Drawing for the job (mm, zero at the part's lowest x, y, z). A direction names the side the tool comes from. Coordinates: 2 decimals unless noted, no trailing zeros. Loops run counter-clockwise (first coordinate to the right, second up) from the corner with the lowest first, then second, coordinate; pieces in that order, holes last. Notation, with made-up numbers: (65, -16.5) -> (76, -16.5) arc R14 cw to (76, -11.5) -> close; hole circle Ø11 at (70.5, 57.5). An arc over 180 degrees is marked (long way). Write each question's results on one line, items separated by ' | '.
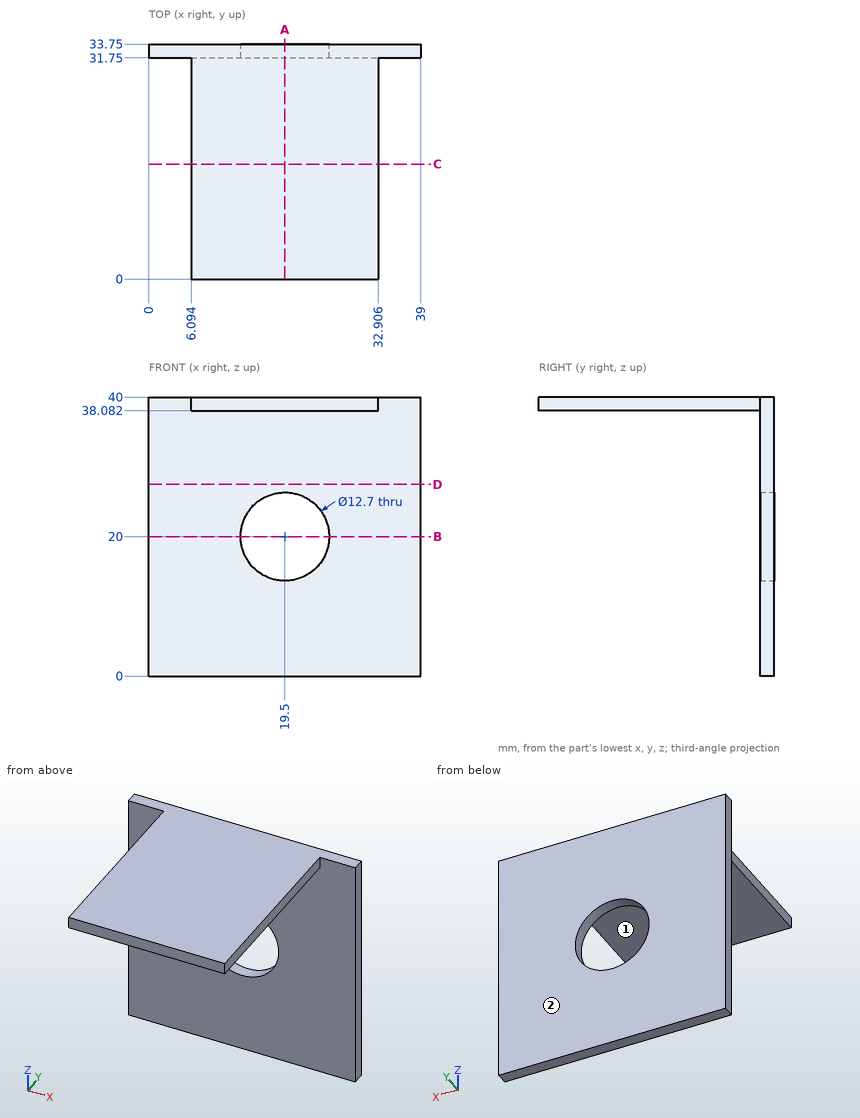
1) Slice it at A-A (x = 19.5). Write the cut outline in (y, z).
Outcome:
outline: (0, 38.08) -> (31.75, 38.08) -> (31.75, 26.35) -> (33.75, 26.35) -> (33.75, 40) -> (0, 40) -> close; (31.75, 0) -> (33.75, 0) -> (33.75, 13.65) -> (31.75, 13.65) -> close
2) Slice it at D-D (z = 27.5). Write the cut outline in (x, y), then the cut area to 3 significant figures.
Outcome:
outline: (0, 31.75) -> (39, 31.75) -> (39, 33.75) -> (0, 33.75) -> close | area: 78.0 mm^2
3) Slice it at C-C (y = 16.5). Write the cut outline in (x, z).
Outcome:
outline: (6.09, 38.08) -> (32.91, 38.08) -> (32.91, 40) -> (6.09, 40) -> close
4) Pin check, flat tips, straight feed: pin 1 (10 mm diameter, centred on y = 28, z = 14, fed in from -X); pin 2 (2 mm diameter, centred on y = 29.5, z = 32, fed in from -X); pin 3 (16.5 mm diameter, centred on x = 19.5, z = 20, fed in from -Y); pin 4 (8 mm diameter, centred on x = 26, y = 15.5, fed in from -Z). Stop position of each tip, or through.
Outcome:
pin 1: stops at x = 0 | pin 2: passes through | pin 3: stops at y = 31.75 | pin 4: stops at z = 38.08
5) Which spindle directions (+Z, -Z, +X, -X, +Y, -Y) get a long thin tool onto all of the face, cutting with end or side? Do the marked faces 1 and 2. Say none if no direction does.
Outcome:
face 1: -Z, +X, -X, -Y | face 2: +Z, -Z, +X, -X, +Y
6) Drill centre lines: L1, parallel to Z at x = 19.5, y = 33.2; L2, parallel to Y at x = 5.5, z = 2.5; L3, parallel to Z at x = 12.5, y = 19. Where is each one in solid material? Low to high. Write a range as from..to.
Outcome:
L1: z = 0..13.65, 26.35..40 | L2: y = 31.75..33.75 | L3: z = 38.08..40
7) Slice it at B-B (z = 20). Write the cut outline in (x, y), then the cut area to 3 significant figures.
Outcome:
outline: (0, 31.75) -> (13.15, 31.75) -> (13.15, 33.75) -> (0, 33.75) -> close; (25.85, 31.75) -> (39, 31.75) -> (39, 33.75) -> (25.85, 33.75) -> close | area: 52.6 mm^2
